Read the model definition and answer for the solid it produces. Units are mm, in the model's axes. Face numbers are marked on the shaded views. A direction names the side the tool comes from. Give positions to 0.01 mm unless a question says otherwise; leave off trailing zeros. Order: outer loops, then holes, each group sorted by start corner. A loop starts at its lowest first (then second) coordinate and runs counter-clockwise, first axis right, second up. Notation, with made-up numbers: (66.25, -30.5) - (90.25, -30.5) arc R21 cw to (90.25, 6.5) - close; hole circle Ø7 at (-34.5, -30). An arc over 180 degrees is marked (long way). Write each question's results on one line, items separated by ' | '. Start each with the question number.
Q1. Flat-ended cylindrical pins translate along their axes: P1, Ø8, axis at x = 9, z = -7.5, coming from the -Y side; P2, Ø1.5, axis at x = 5.5, y = -0.5, coming from the -Z side (3 decimals); P3, Ø5, axis at x = 12, y = 3, coming from the +Z side. Find the tip coordinate at first contact, or state that the pin passes through.
Q2. Find section A-A on z = 0. Give the vertices of the cut face in (x, y).
Q3. Find section D-D on x = -1.5. Give the vertices of the cut face in (y, z) (3 decimals), and give its area (3 significant figures).
Q4. Find section C-C on x = 13.25. Give the vertices of the cut face in (y, z) (1 decimal), and give its area (3 significant figures).
Q5. Find section B-B on y = -3.75. Give the vertices of the cut face in (x, z) (3 decimals).
Q6. A tool of negligible diameter and unlimited length cuts with its end or side. For the marked faces 1, 2, 3, 4 and 5, from which of +Z, -Z, +X, -X, +Y, -Y can it reach the whole face along a straight path? Write none if from no direction.
Q7. For a pull along Y with two mould halves and no side action, classify the marked faces 6, 7 and 8 as +Y half, -Y half, draft (parallel to the pull), parting line (faces both ways), or undercut.
Q8. Find the intervals of material crossed by line 1 along Y through (x, z) = (14, 0); line 2 along Z through (x, y) = (3, -2.25) (3 decimals); line 3 along Z through (x, y) = (16, -1.5), in increasing order. Write a range as from..to.
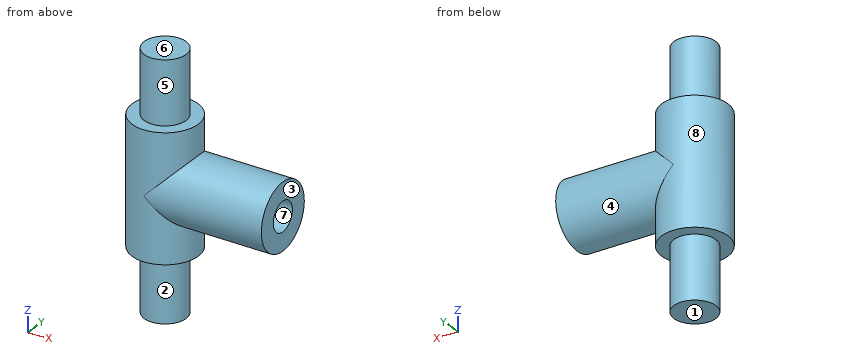
from build123d import *

# Parameters (mm, degrees)
SKETCH1_R           = 5
BOSS_EXTRUDE1_DEPTH = 9.525
SKETCH5_R           = 3.175
BOSS_EXTRUDE4_DEPTH = 19.05
SKETCH6_R           = 5
BOSS_EXTRUDE5_DEPTH = 17.78
SKETCH7_R           = 2.2225
CUT_EXTRUDE1_DEPTH  = 12.7


with BuildPart() as part:
    # Sketch1 → Boss-Extrude1 (new, symmetric)
    with BuildSketch(Plane.XY):
        with Locations(Location((0, 0, 0), (0, 0, 180))):
            Circle(SKETCH1_R)
    extrude(amount=BOSS_EXTRUDE1_DEPTH, both=True)

    # Sketch5 → Boss-Extrude4 (add, symmetric)
    with BuildSketch(Plane.XY):
        with Locations(Location((0, 0, 0), (0, 0, 180))):
            Circle(SKETCH5_R)
    extrude(amount=BOSS_EXTRUDE4_DEPTH, both=True)

    # Sketch6 → Boss-Extrude5 (add)
    with BuildSketch(Plane(origin=(0, 0, 0), x_dir=(0, 0, -1), z_dir=(1, 0, 0))):
        Circle(SKETCH6_R)
    extrude(amount=BOSS_EXTRUDE5_DEPTH)

    # Sketch7 → Cut-Extrude1 (cut)
    with BuildSketch(Plane(origin=(17.78, 0, 0), x_dir=(0, 0, -1), z_dir=(1, 0, 0))):
        Circle(SKETCH7_R)
    extrude(amount=-CUT_EXTRUDE1_DEPTH, mode=Mode.SUBTRACT)


solid = part.part
Working result:
1) P1: y = -3.57 | P2: z = -9.525 | P3: z = 4.97
2) outline: (0, -5) - (17.78, -5) - (17.78, -2.22) - (5.08, -2.22) - (5.08, 2.22) - (17.78, 2.22) - (17.78, 5) - (0, 5) arc R5 ccw to start
3) outline: (-4.77, -9.525) - (-2.798, -9.525) - (-2.798, -19.05) - (2.798, -19.05) - (2.798, -9.525) - (4.77, -9.525) - (4.77, 9.525) - (2.798, 9.525) - (2.798, 19.05) - (-2.798, 19.05) - (-2.798, 9.525) - (-4.77, 9.525) - close | area: 288 mm²
4) outline: circle Ø10 at (0, 0); hole circle Ø4.4 at (0, 0) | area: 63.0 mm²
5) outline: (-3.307, -9.525) - (3.307, -9.525) - (3.307, -3.307) - (17.78, -3.307) - (17.78, 3.307) - (3.307, 3.307) - (3.307, 9.525) - (-3.307, 9.525) - close
6) face 1: -Z, +X, -X, +Y, -Y | face 2: -Z | face 3: +Z, -Z, +X, +Y, -Y | face 4: +X | face 5: +Z
7) face 6: draft | face 7: undercut | face 8: parting line
8) line 1: -5..-2.22, 2.22..5 | line 2: -9.525..9.525 | line 3: -4.77..-1.64, 1.64..4.77
